Can you work these out from the model? Positions are in its coordinate system, mm. A direction names the side the tool comes from. Coordinates: 2 decimals unless noted, no trailing zeros. Loops run counter-clockwise (first coordinate to the right, second up) from the corner with the lowest first, then second, coordinate; pieces in that order, holes last.
```python
from build123d import *

# Parameters (mm, degrees)
BOSS_EXTRUDE1_DEPTH = 9.525
SKETCH3_R           = 1.55
CUT_EXTRUDE2_DEPTH  = 5.08
SKETCH4_R           = 1.55
CUT_EXTRUDE3_DEPTH  = 5.08
CIRPATTERN2_COUNT   = 3


with BuildPart() as part:
    # Sketch1 → Boss-Extrude1 (new body)
    with BuildSketch(Plane.XY):
        with BuildLine():
            Line((12.7, 21.969079793), (12.7, 43.5864))
            ThreePointArc((12.7, 43.5864), (11.584076836, 46.280476836), (8.89, 47.3964))
            Line((8.89, 47.3964), (-8.89, 47.3964))
            ThreePointArc((-8.89, 47.3964), (-11.584076836, 46.280476836), (-12.7, 43.5864))
            Line((-12.7, 43.5864), (-12.7, 21.969079793))
            ThreePointArc((-12.7, 21.969079793), (-13.101409662, 20.266842468), (-14.221056121, 18.923289925))
            ThreePointArc((-14.221056121, 18.923289925), (-20.499926929, 11.835638331), (-23.498577859, 2.854150907))
            ThreePointArc((-23.498577859, 2.854150907), (-24.102305263, 1.212732359), (-25.375781199, 0.013982731))
            Line((-25.375781199, 0.013982731), (-44.09692966, -10.794677372))
            ThreePointArc((-44.09692966, -10.794677372), (-45.872107058, -13.108133599), (-45.491486448, -15.99923416))
            Line((-45.491486448, -15.99923416), (-36.601486448, -31.39716584))
            ThreePointArc((-36.601486448, -31.39716584), (-34.288030221, -33.172343238), (-31.39692966, -32.791722628))
            Line((-31.39692966, -32.791722628), (-12.675781199, -21.983062525))
            ThreePointArc((-12.675781199, -21.983062525), (-11.000895601, -21.479574827), (-9.277521738, -21.777440832))
            ThreePointArc((-9.277521738, -21.777440832), (0, -23.671276662), (9.277521738, -21.777440832))
            ThreePointArc((9.277521738, -21.777440832), (11.000895601, -21.479574827), (12.675781199, -21.983062525))
            Line((12.675781199, -21.983062525), (31.39692966, -32.791722628))
            ThreePointArc((31.39692966, -32.791722628), (34.288030221, -33.172343238), (36.601486448, -31.39716584))
            Line((36.601486448, -31.39716584), (45.491486448, -15.99923416))
            ThreePointArc((45.491486448, -15.99923416), (45.872107058, -13.108133599), (44.09692966, -10.794677372))
            Line((44.09692966, -10.794677372), (25.375781199, 0.013982731))
            ThreePointArc((25.375781199, 0.013982731), (24.102305263, 1.212732359), (23.498577859, 2.854150907))
            ThreePointArc((23.498577859, 2.854150907), (20.499926929, 11.835638331), (14.221056121, 18.923289925))
            ThreePointArc((14.221056121, 18.923289925), (13.101409662, 20.266842468), (12.7, 21.969079793))
        make_face()
    extrude(amount=BOSS_EXTRUDE1_DEPTH)

    # Sketch3 → Cut-Extrude2 (cut)
    with BuildSketch(Plane(origin=(-6.35, -10.998522628, 0), x_dir=(0.866025404, -0.5, 0), z_dir=(-0.5, -0.866025404, 0))):
        with Locations((39.7764, 3.582)):
            Circle(SKETCH3_R)
    cut_extrude2 = extrude(amount=-CUT_EXTRUDE2_DEPTH, mode=Mode.SUBTRACT)

    # Sketch4 → Cut-Extrude3 (cut)
    with BuildSketch(Plane(origin=(6.35, 10.998522628, 0), x_dir=(0.866025404, -0.5, 0), z_dir=(0.5, 0.866025404, 0))):
        with Locations((39.7764, -3.582)):
            Circle(SKETCH4_R)
    cut_extrude3 = extrude(amount=-CUT_EXTRUDE3_DEPTH, mode=Mode.SUBTRACT)

    # CirPattern2: Cut-Extrude2, Cut-Extrude3 ×3 about axis
    cirpattern2_axis = Axis((0, 0, 0), (0, 0, 1))
    for i in range(1, CIRPATTERN2_COUNT):
        add(cut_extrude2.rotate(cirpattern2_axis, i * 360 / CIRPATTERN2_COUNT), mode=Mode.SUBTRACT)
        add(cut_extrude3.rotate(cirpattern2_axis, i * 360 / CIRPATTERN2_COUNT), mode=Mode.SUBTRACT)


solid = part.part
```
Item 1: Suppose I cut it at C-C, the plane x = 1. Please give me the cut outline in (y, z) (3 decimals), plus the area to 3 significant figures.
Results are:
outline: (-23.65, 0) - (47.396, 0) - (47.396, 9.525) - (-23.65, 9.525) - close
area: 677 mm2
Item 2: Suppose I cut it at B-B, the plane y = 8. Please give me the cut outline in (x, z) (3 decimals), plus the area to 3 significant figures.
Results are:
outline: (-22.278, 0) - (22.278, 0) - (22.278, 9.525) - (-22.278, 9.525) - close
area: 424 mm2
Item 3: I need wall thicknesses on line 1 along Y through (x, z) = (38, 3.5); line 2 along Y through (x, z) = (-1, 2); line 3 along X through (y, z) = (33, 1). Which ranges of each line are inside material? Lowest first, please.
Results are:
line 1: y = -28.97 to -13.14, -10.64 to -7.27
line 2: y = -23.65 to 47.4
line 3: x = -12.7 to 12.7
Item 4: On a 3-axis mill with a long thin cutter (end or side, diameter ignored), from which of +Z, -Z, +X, -X, +Y, -Y can I reach the whole of each face in a straight line? I mean faces 1 (the face through (-10.196, 40.61, 2.275)), 2 (the face through (7.62, 40, 4)), 3 (the face through (21.905, -27.312, 4.696)), 4 (the face through (30.619, -26.476, 3.604)). Say none if no direction works.
Results are:
face 1: -X
face 2: +X
face 3: +Z, -Z, -Y
face 4: none
Item 5: We'd pull the mould along Y, two halves only. Please class faces 5 (the face through (-30.59, -29.43, 4.18)), 6 (the face through (20.566, 11.72, 4.696)), 7 (the face through (-0.13, -23.67, 4.7)): +Y half, -Y half, draft (parallel to the pull), parting line (faces both ways), or undercut.
Results are:
face 5: undercut
face 6: +Y half
face 7: -Y half
Item 6: I'm going to push flat-ended pins straight in: P1, Ø1, axis at x = 29, z = 4, coming from the +Y side; P2, Ø3, axis at y = 38, z = 4, coming from the -X side; P3, Ø4, axis at y = 39.78, z = 3.58, coming from the +X side. Where does each tip first touch, or does it pass through?
Results are:
P1: stops at y = -1.79
P2: stops at x = -12.7
P3: stops at x = 12.7
Item 7: Suppose I cut it at A-A, the plane z = 6.75. Please give me the cut outline in (x, y), plus the area to 3 significant figures.
Results are:
outline: (-45.49, -16) - (-36.6, -31.4) arc R3.81 ccw to (-31.4, -32.79) - (-12.68, -21.98) arc R3.81 cw to (-9.28, -21.78) arc R23.67 ccw to (9.28, -21.78) arc R3.81 cw to (12.68, -21.98) - (31.4, -32.79) arc R3.81 ccw to (36.6, -31.4) - (45.49, -16) arc R3.81 ccw to (44.1, -10.79) - (25.38, 0.01) arc R3.81 cw to (23.5, 2.85) arc R23.67 ccw to (14.22, 18.92) arc R3.81 cw to (12.7, 21.97) - (12.7, 43.59) arc R3.81 ccw to (8.89, 47.4) - (-8.89, 47.4) arc R3.81 ccw to (-12.7, 43.59) - (-12.7, 21.97) arc R3.81 cw to (-14.22, 18.92) arc R23.67 ccw to (-23.5, 2.85) arc R3.81 cw to (-25.38, 0.01) - (-44.1, -10.79) arc R3.81 ccw to start
area: 3,640 mm2
